from build123d import *

# Parameters (mm, degrees)
ESBO_O1_W                = 64
ESBO_O1_H                = 64
ESBO_O1_R                = 2
RESSALTO_EXTRUS_O1_DEPTH = 5
ESBO_O2_W                = 64
ESBO_O2_H                = 5
RESSALTO_EXTRUS_O3_DEPTH = 80
ESBO_O3_R                = 11
ESBO_O3_R_2              = 2
CORTE_EXTRUS_O1_DEPTH    = 114


with BuildPart() as part:
    # Esboço1 → Ressalto-extrusão1 (new body)
    with BuildSketch(Plane.XY):
        with Locations((32, 32)):
            Rectangle(ESBO_O1_W, ESBO_O1_H)
        with Locations((32, 42.5)):
            Circle(ESBO_O1_R, mode=Mode.SUBTRACT)
        with Locations((32, 32)):
            Circle(ESBO_O1_R, mode=Mode.SUBTRACT)
        with Locations((32, 21.5)):
            Circle(ESBO_O1_R, mode=Mode.SUBTRACT)
        with Locations((32, 53)):
            Circle(ESBO_O1_R, mode=Mode.SUBTRACT)
        with Locations((32, 11)):
            Circle(ESBO_O1_R, mode=Mode.SUBTRACT)
    extrude(amount=RESSALTO_EXTRUS_O1_DEPTH)

    # Esboço2 → Ressalto-extrusão3 (add)
    with BuildSketch(Plane.XY):
        with Locations((32, 50)):
            Rectangle(ESBO_O2_W, ESBO_O2_H)
    extrude(amount=RESSALTO_EXTRUS_O3_DEPTH)

    # Esboço3 → Corte-extrusão1 (cut)
    with BuildSketch(Plane(origin=(0, 0, 0), x_dir=(1, 0, 0), z_dir=(0, 1, 0))):
        with Locations((32, -59)):
            Circle(ESBO_O3_R)
        with Locations((15.45, -74)):
            Circle(ESBO_O3_R_2)
        with Locations((48.55, -74)):
            Circle(ESBO_O3_R_2)
        with Locations((15.45, -44)):
            Circle(ESBO_O3_R_2)
        with Locations((48.55, -44)):
            Circle(ESBO_O3_R_2)
        with Locations((7.003644385, -20)):
            Circle(ESBO_O3_R_2)
        with Locations((57.465770744, -20)):
            Circle(ESBO_O3_R_2)
    extrude(amount=CORTE_EXTRUS_O1_DEPTH, mode=Mode.SUBTRACT)


solid = part.part
Model file for the job. Use its own axes, mm. A direction names the side the tool comes from. Round coordinates to 2 decimals unless told otherwise and drop trailing zeros. Order: outer loops, then holes, each group sorted by start corner. A loop starts at its lowest first (then second) coordinate and runs counter-clockwise, first axis right, second up. Notation, with made-up numbers: M 78,-5.5 L 104,-5.5 A25 ccw 104,28.5 Z; hole C 65.5,3.5 d10. An arc over 180 degrees is marked long. Write each question's results on one line, items separated by ' | '. Start each with the question number.
(1) Drop flat-ended pins along their axis: pin 1 (5 mm diameter, centred on x = 48.55, z = 74, fed in from -Y); pin 2 (5 mm diameter, centred on x = 32, y = 53, fed in from -Z); pin 3 (10 mm diameter, centred on x = 51, z = 22, fed in from +Y). Give the stop position or say it passes through.
(2) Saw through at A-A, the plane z = 59. Give the cut face in (x, y).
(3) Saw through at B-B, the plane y = 48.5. Give the cut face in (x, z).
(4) Saw through at C-C, the plane z = 74. Give the cut face in (x, y).
(5) Saw through at D-D, the plane x = 37. Give the cut face in (y, z).
(6) Probe probe 1 along Y at (x, z) = (32, 3.2); probe 2 along Z at (x, y) = (16.5, 59); probe 3 along Z at (x, y) = (48, 51). List the from-to ranges inside material, lowest first. Write a range as from..to.
(7) Which spindle directions (+Z, -Z, +X, -X, +Y, -Y) get a long thin tool onto all of the face, cutting with end or side? Do faces 1 (the face through (32, 58, 5)), 2 (the face through (32.923, 40.726, 2.465)), 3 (the face through (32, 47.5, 42)). Say none if no direction does.
(8) Two-plate mould, pull along Z, no slides. Class faces 4 (the face through (32, 0, 2)), 5 (the face through (32, 50, 80)), 6 (the face through (42.492, 49.965, 55.696)): pulls with the +Z half, pulls with the -Z half, needs draft (parallel to the pull), parting line crosses it, or undercut.
Established:
1) pin 1: stops at y = 47.5 | pin 2: stops at z = 0 | pin 3: stops at y = 52.5
2) outline: M 0,47.5 L 21,47.5 L 21,52.5 L 0,52.5 Z; M 43,47.5 L 64,47.5 L 64,52.5 L 43,52.5 Z
3) outline: M 0,0 L 64,0 L 64,80 L 0,80 Z; hole C 7,20 d4; hole C 15.45,44 d4; hole C 15.45,74 d4; hole C 32,59 d22; hole C 48.55,44 d4; hole C 48.55,74 d4; hole C 57.47,20 d4
4) outline: M 0,47.5 L 13.45,47.5 L 13.45,52.5 L 0,52.5 Z; M 17.45,47.5 L 46.55,47.5 L 46.55,52.5 L 17.45,52.5 Z; M 50.55,47.5 L 64,47.5 L 64,52.5 L 50.55,52.5 Z
5) outline: M 0,0 L 64,0 L 64,5 L 52.5,5 L 52.5,49.2 L 47.5,49.2 L 47.5,5 L 0,5 Z; M 47.5,68.8 L 52.5,68.8 L 52.5,80 L 47.5,80 Z
6) probe 1: y = 0..9, 13..19.5, 23.5..30, 34..40.5, 44.5..52.5, 55..64 | probe 2: z = 0..5 | probe 3: z = 0..42.08, 45.92..72.08, 75.92..80
7) face 1: +Z, +X, -X, +Y | face 2: +Z, -Z | face 3: +Z, +X, -X, -Y
8) face 4: needs draft | face 5: pulls with the +Z half | face 6: undercut
